Can you work these out from the model? Positions are in its coordinate system, mm. A direction names the side the tool comes from. Give positions to 0.01 mm unless a question says otherwise; leave off trailing zeros. Order: outer loops, then holes, each group sorted by start corner. A loop starts at its lowest first (then second) coordinate and runs counter-clockwise, first axis right, second up. Notation, with made-up numbers: (67.25, 63.5) - (90.25, 63.5) arc R29 ccw to (90.25, 95.5) - close; hole circle Ø9 at (3.25, 49). An arc over 180 degrees is marked (long way). Return JSON: item names as keys, results as strings.
```python
from build123d import *

# Parameters (mm, degrees)
F0_W     = 80
F0_H     = 120
F0_W_2   = 10
F0_H_2   = 50
F0_W_3   = 30
F0_H_3   = 10
F1_DEPTH = 5


with BuildPart() as f1:
    # F0 (on Right) → F1 (new body)
    with BuildSketch(Plane.YZ):
        Rectangle(F0_W, F0_H)
        Polygon((35, -5), (35, -55), (5, -55), (-5, -55), (-35, -55), (-35, -5), (-35, 5), (-35, 55), (-5, 55), (5, 55), (35, 55), (35, 5), align=None, mode=Mode.SUBTRACT)
        with Locations((0, -30)):
            Rectangle(F0_W_2, F0_H_2)
        with Locations((0, 30)):
            Rectangle(F0_W_2, F0_H_2)
        with Locations((-20, 0)):
            Rectangle(F0_W_3, F0_H_3)
        with Locations((20, 0)):
            Rectangle(F0_W_3, F0_H_3)
        Rectangle(F0_W_2, F0_H_3)
    extrude(amount=F1_DEPTH)


solid = f1.part
```
1. If I drill on L1, parallel to Y at x = 1.4, z = -24.5; L2, parallel to Z at x = 2.4, y = 16.5, over which ranges is the centre line in solid material (lowest first)? Write a range as [from, to].
Checks:
{"L1": "[-40, -35], [-5, 5], [35, 40]", "L2": "[-60, -55], [-5, 5], [55, 60]"}
2. Thinking about a two-plate mould opening in Z: for faces 1 (the face through (2, -35, -30)), 2 (the face through (2, 40, -1)), which applies, +Z half, -Z half, draft (parallel to the pull), parting line (faces both ways), or undercut?
Checks:
{"face 1": "undercut", "face 2": "draft"}
3. Suppose I cut it at B-B (y = -29). List the corners of the cut face in (x, z) for me.
Checks:
{"outline": "(0, -60) - (5, -60) - (5, -55) - (0, -55) - close; (0, -5) - (5, -5) - (5, 5) - (0, 5) - close; (0, 55) - (5, 55) - (5, 60) - (0, 60) - close"}
4. On a 3-axis mill with a long thin cutter (end or side, diameter ignored), from which of +Z, -Z, +X, -X, +Y, -Y can I reach the whole of each face in a straight line? I mean faces 3 (the face through (2, 35, 30)), 4 (the face through (5, 3, 0)). Say none if no direction works.
Checks:
{"face 3": "+X, -X", "face 4": "+Z, -Z, +X, +Y, -Y"}
5. Suppose I cut it at C-C (x = 3.85). List the corners of the cut face in (y, z) for me, plus the area to 3 significant figures.
Checks:
{"outline": "(-40, -60) - (40, -60) - (40, 60) - (-40, 60) - close; hole (-35, -55) - (-5, -55) - (-5, -5) - (-35, -5) - close; hole (-35, 5) - (-5, 5) - (-5, 55) - (-35, 55) - close; hole (5, -55) - (35, -55) - (35, -5) - (5, -5) - close; hole (5, 5) - (35, 5) - (35, 55) - (5, 55) - close", "area": "3,600 mm^2"}
6. Suppose I cut it at A-A (z = -42). List the corners of the cut face in (x, y) for me, plus the area to 3 significant figures.
Checks:
{"outline": "(0, -40) - (5, -40) - (5, -35) - (0, -35) - close; (0, -5) - (5, -5) - (5, 5) - (0, 5) - close; (0, 35) - (5, 35) - (5, 40) - (0, 40) - close", "area": "100 mm^2"}
